Design review of the part built by this model. Coordinates are the model's own, in mm. Face numbers are marked on the shaded views. A direction names the side the tool comes from. Coordinates: 2 decimals unless noted, no trailing zeros. Loops run counter-clockwise (first coordinate to the right, second up) from the corner with the lowest first, then second, coordinate; pieces in that order, holes last. Notation, with made-up numbers: (81.25, -38) -> (90.25, -38) arc R8 ccw to (90.25, -30) -> close; hole circle Ø11 at (79.25, -23). An arc over 180 degrees is marked (long way). Answer as a JSON object with one key per item and string values.
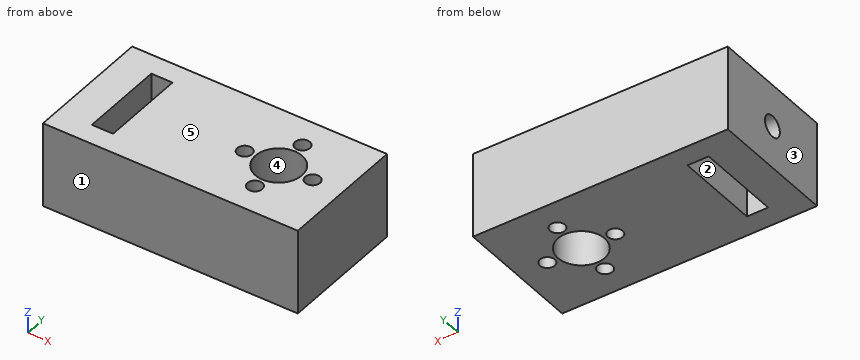
```python
from build123d import *

# Parameters (mm, degrees)
SKETCH1_W           = 60
SKETCH1_H           = 30
SKETCH1_R           = 5.5
SKETCH1_R_2         = 1.75
SKETCH1_W_2         = 5
SKETCH1_H_2         = 20
BOSS_EXTRUDE1_DEPTH = 10
SKETCH2_R           = 2.5
CUT_EXTRUDE1_DEPTH  = 8


with BuildPart() as part:
    # Sketch1 → Boss-Extrude1 (new, symmetric)
    with BuildSketch(Plane.XY):
        Rectangle(SKETCH1_W, SKETCH1_H)
        with Locations((15, 0)):
            Circle(SKETCH1_R, mode=Mode.SUBTRACT)
        with Locations((15, 8)):
            Circle(SKETCH1_R_2, mode=Mode.SUBTRACT)
        with Locations((23, 0)):
            Circle(SKETCH1_R_2, mode=Mode.SUBTRACT)
        with Locations((15, -8)):
            Circle(SKETCH1_R_2, mode=Mode.SUBTRACT)
        with Locations((7, 0)):
            Circle(SKETCH1_R_2, mode=Mode.SUBTRACT)
        with Locations((-19.5, 0)):
            Rectangle(SKETCH1_W_2, SKETCH1_H_2, mode=Mode.SUBTRACT)
    extrude(amount=BOSS_EXTRUDE1_DEPTH, both=True)

    # Sketch2 → Cut-Extrude1 (cut)
    with BuildSketch(Plane.ZY.offset(30)):
        with Locations(Location((0, 0, 0), (0, 0, 270))):
            Circle(SKETCH2_R)
    extrude(amount=-CUT_EXTRUDE1_DEPTH, mode=Mode.SUBTRACT)


solid = part.part
```
1) Add section A-A, the plane y = 8. Give the boundary of the cut face in (x, z).
Completed:
{"outline": "(-30, -10) -> (-22, -10) -> (-22, 10) -> (-30, 10) -> close; (-17, -10) -> (13.25, -10) -> (13.25, 10) -> (-17, 10) -> close; (16.75, -10) -> (30, -10) -> (30, 10) -> (16.75, 10) -> close"}
2) Wall thickness on probe 1 along Y at (x, z) = (15, 5.25); probe 2 along Y at (x, z) = (16, -7); probe 3 along X at (y, z) = (8.75, 2.25): over which ranges is each line inside the solid? List them lowest first.
Completed:
{"probe 1": "-15 to -9.75, -6.25 to -5.5, 5.5 to 6.25, 9.75 to 15", "probe 2": "-15 to -9.44, -6.56 to -5.41, 5.41 to 6.56, 9.44 to 15", "probe 3": "-30 to -22, -17 to 13.42, 16.58 to 30"}
3) For the marked faces 1 and 2, list the 3-axis set-ups (+Z, -Z, +X, -X, +Y, -Y) from which the entire face can be reached by the end or side of a thin tool; tool diameter is ignored.
Completed:
{"face 1": "+Z, -Z, +X, -X, -Y", "face 2": "+Z, -Z"}
4) Add section C-C, the plane x = 7. Give the boundary of the cut face in (y, z).
Completed:
{"outline": "(-15, -10) -> (-1.75, -10) -> (-1.75, 10) -> (-15, 10) -> close; (1.75, -10) -> (15, -10) -> (15, 10) -> (1.75, 10) -> close"}
5) Add section B-B, the plane x = 15. Give the boundary of the cut face in (y, z).
Completed:
{"outline": "(-15, -10) -> (-9.75, -10) -> (-9.75, 10) -> (-15, 10) -> close; (-6.25, -10) -> (-5.5, -10) -> (-5.5, 10) -> (-6.25, 10) -> close; (5.5, -10) -> (6.25, -10) -> (6.25, 10) -> (5.5, 10) -> close; (9.75, -10) -> (15, -10) -> (15, 10) -> (9.75, 10) -> close"}
6) The part is to be moulded in two halves that separate along X. For the marked faces 3, 4 and 5, say which applies: pulls with the +X half, pulls with the -X half, needs draft (parallel to the pull), parting line crosses it, or undercut.
Completed:
{"face 3": "pulls with the -X half", "face 4": "undercut", "face 5": "needs draft"}
7) Add section D-D, the plane z = 0. Give the boundary of the cut face in (x, y), and give its area (3 significant figures).
Completed:
{"outline": "(-30, -15) -> (30, -15) -> (30, 15) -> (-30, 15) -> (-30, 2.5) -> (-22, 2.5) -> (-22, 10) -> (-17, 10) -> (-17, -10) -> (-22, -10) -> (-22, -2.5) -> (-30, -2.5) -> close; hole circle Ø3.5 at (7, 0); hole circle Ø11 at (15, 0); hole circle Ø3.5 at (15, -8); hole circle Ø3.5 at (15, 8); hole circle Ø3.5 at (23, 0)", "area": "1,530 mm²"}
